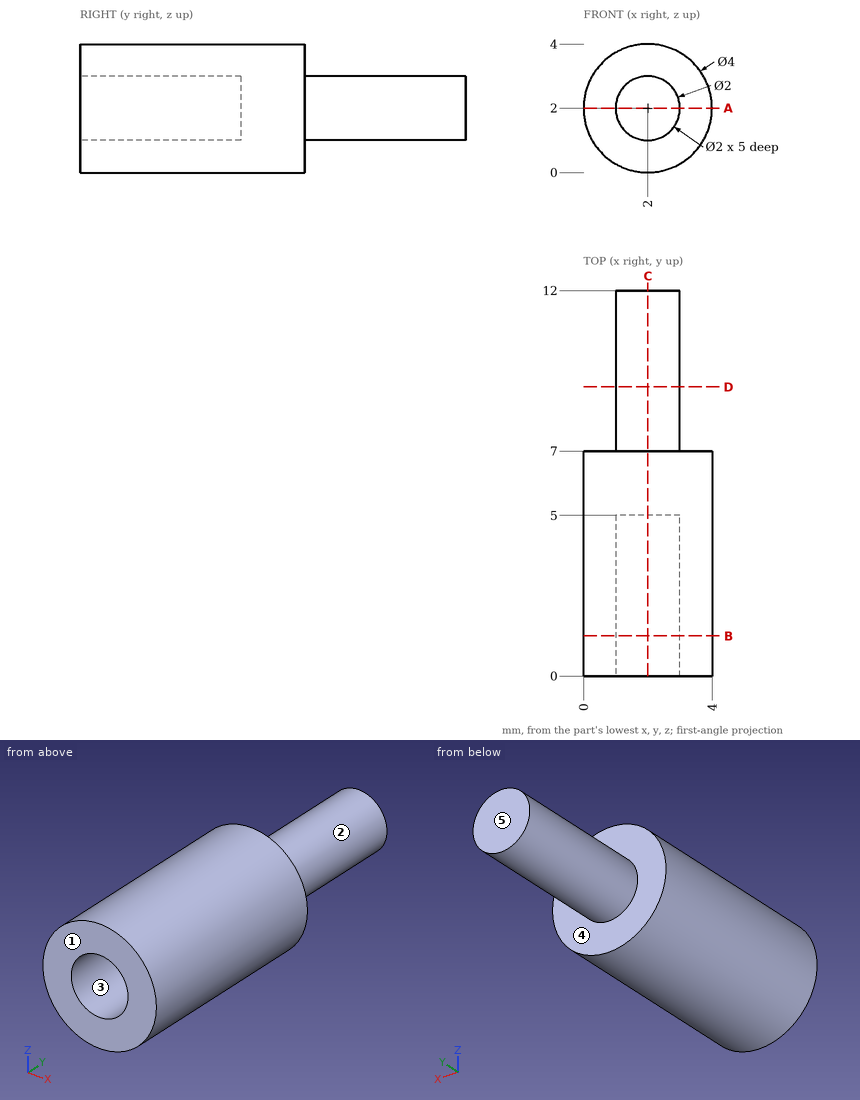
Verification items for this drawing (mm, ordinates from the low corner). A direction names the side the tool comes from. Round coordinates to 2 decimals unless told otherwise and drop trailing zeros. Loops run counter-clockwise (first coordinate to the right, second up) from the corner with the lowest first, then second, coordinate; pieces in that order, holes last. Notation, with made-up numbers: (58, 17) -> (107, 17) arc R16 ccw to (107, 23) -> close; hole circle Ø1 at (-3, -14.5). An arc over 180 degrees is marked (long way). Write item = value, one per line. Start each with the question number.
1) Thickness scan on probe 1 along Z at (x, y) = (2, 3.2); probe 2 along Y at (x, z) = (2.35, 2.8); probe 3 along Y at (x, z) = (1.85, 0.55). Record the ranges inside material, lowest first.
2) Release check for a two-part mould opening along X. For the marked faces 1, 2 and 3 record: released by +X, released by -X, zero draft, split by the parting line, or undercut.
3) Sectioned sample at B-B, the plane y = 1.25. Record the cut outline in (x, z), plus the area to 3 significant figures.
4) Sectioned sample at D-D, the plane y = 9. Record the cut outline in (x, z).
5) Sectioned sample at A-A, the plane z = 2. Record the cut outline in (x, y), plus the area to 3 significant figures.
6) Sectioned sample at C-C, the plane x = 2. Record the cut outline in (y, z).
7) Gauge pin test, flat ends, axial feed: pin 1 Ø2 at (x, y) = (3.5, 3) entering from -Z; pin 2 Ø1.5 at (x, y) = (1, 8) entering from +Z; pin 3 Ø1 at (x, z) = (2, 2) entering from -Y. Record the tip position at first contact, or that the pin passes through.
8) Set-up check for the marked faces 4 and 5: record each of +Z, -Z, +X, -X, +Y, -Y from which the full face is reachable in a straight line by a thin tool's end or side.
Results are:
q1.probe_1 = 0 to 1, 3 to 4
q1.probe_2 = 5 to 12
q1.probe_3 = 0 to 7
q2.face_1 = zero draft
q2.face_2 = split by the parting line
q2.face_3 = undercut
q3.outline = circle Ø4 at (2, 2); hole circle Ø2 at (2, 2)
q3.area = 9.42 mm^2
q4.outline = circle Ø2 at (2, 2)
q5.outline = (0, 0) -> (1, 0) -> (1, 5) -> (3, 5) -> (3, 0) -> (4, 0) -> (4, 7) -> (3, 7) -> (3, 12) -> (1, 12) -> (1, 7) -> (0, 7) -> close
q5.area = 28.0 mm^2
q6.outline = (0, 0) -> (7, 0) -> (7, 1) -> (12, 1) -> (12, 3) -> (7, 3) -> (7, 4) -> (0, 4) -> (0, 3) -> (5, 3) -> (5, 1) -> (0, 1) -> close
q7.pin_1 = 0.06
q7.pin_2 = 2.97
q7.pin_3 = 5
q8.face_4 = +Y
q8.face_5 = +Z, -Z, +X, -X, +Y
